from build123d import *

# Parameters (mm, degrees)
BOSS_EXTRUDE2_DEPTH = 5
CUT_EXTRUDE1_REACH  = 24.845
SKETCH3_R           = 2.1
CUT_EXTRUDE2_START  = -1.2
CUT_EXTRUDE2_DEPTH  = 3.6


with BuildPart() as part:
    # Sketch1 → Boss-Extrude2 (new body)
    with BuildSketch(Plane(origin=(0, 0, 0), x_dir=(1, 0, 0), z_dir=(0, 1, 0))):
        with BuildLine():
            Line((-0.939692556, 20.223890242), (-7.329602442, 2.667757118))
            ThreePointArc((-7.329602442, 2.667757118), (0, -7.8), (7.329602442, 2.667757118))
            Line((7.329602442, 2.667757118), (0.939692556, 20.223890242))
            ThreePointArc((0.939692556, 20.223890242), (0, 20.881870053), (-0.939692556, 20.223890242))
        make_face()
    extrude(amount=BOSS_EXTRUDE2_DEPTH)

    # Sketch3 → Cut-Extrude1 (cut, up to next)
    with BuildSketch(Plane(origin=(0, 5, 0), x_dir=(1, 0, 0), z_dir=(0, 1, 0)), mode=Mode.PRIVATE) as cut_extrude1_sk1:
        with Locations(Location((0, 0, 0), (0, 0, 270))):
            Circle(SKETCH3_R)
    cut_extrude1_tool1 = extrude(cut_extrude1_sk1.sketch, amount=-CUT_EXTRUDE1_REACH, mode=Mode.PRIVATE) & part.part
    add(cut_extrude1_tool1.solids().sort_by_distance((0, 5, 0))[0], mode=Mode.SUBTRACT)

    # Sketch4 → Cut-Extrude2 (cut)
    with BuildSketch(Plane(origin=(0, 5, 0), x_dir=(1, 0, 0), z_dir=(0, 1, 0)).offset(CUT_EXTRUDE2_START)):
        Polygon((0, 4.272391992), (-3.7, 2.136195996), (-3.7, -2.136195996), (0, -4.272391992), (3.7, -2.136195996), (3.7, 2.136195996), align=None)
    extrude(amount=-CUT_EXTRUDE2_DEPTH, mode=Mode.SUBTRACT)


solid = part.part
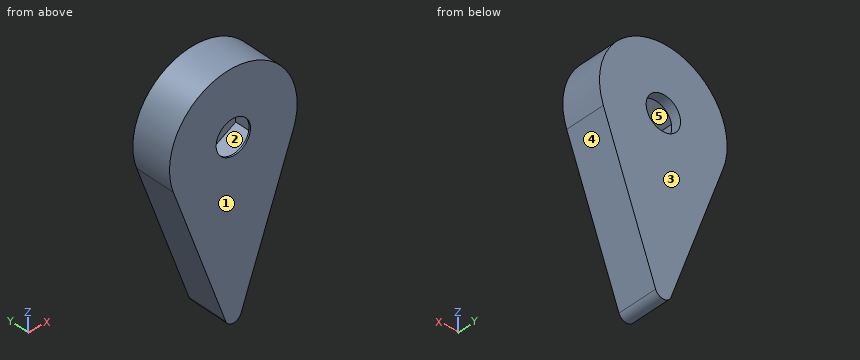
Work out the finished part from the listing and answer in its coordinate system (mm). Face numbers are marked on the shaded views. A direction names the side the tool comes from. Give positions to 0.01 mm unless a question says otherwise; leave off trailing zeros. Write each loop counter-clockwise with the first axis right and the second up, starting at its lowest first coordinate (ties: lowest second). Pieces come first, ordered by that corner, then holes. Notation, with made-up numbers: M -16.75,61.25 L 40.25,61.25 A22 ccw 40.25,78.25 Z; hole C 48,32.25 d3. An arc over 180 degrees is marked long. Answer as CSV lines item,"result".
Q1. A tool of negligible diameter and unlimited length cuts with its end or side. For the marked faces 1 and 2, from which of +Z, -Z, +X, -X, +Y, -Y can it reach the whole face along a straight path? Write none if from no direction.
A:
face 1,"+Z, -Z, +X, -X, -Y"
face 2,"none"
Q2. A cutting plane is placed at D-D on y = 4.6. Write down the section's boundary in (x, z).
A:
outline,"M -7.33,-2.67 L -0.94,-20.22 A1 ccw 0.94,-20.22 L 7.33,-2.67 A7.8 ccw long Z; hole C 0,0 d4.2"
Q3. Given P1, Ø4, axis at x = 0, z = 0, coming from the -Y side; P2, Ø2, axis at x = -4.5, y = 1.5, coming from the +Z side, each flat-ended and moving along its own axis, determine where each tip first touches the part or whether it passes through.
A:
P1,"passes through"
P2,"stops at z = 6.97"
Q4. A cutting plane is placed at C-C on x = 1.5. Write down the section's boundary in (y, z).
A:
outline,"M 0,-18.68 L 5,-18.68 L 5,-1.47 L 3.8,-1.47 L 3.8,-3.41 L 0.2,-3.41 L 0.2,-1.47 L 0,-1.47 Z; M 0,1.47 L 0.2,1.47 L 0.2,3.41 L 3.8,3.41 L 3.8,1.47 L 5,1.47 L 5,7.65 L 0,7.65 Z"
Q5. A cutting plane is placed at B-B on z = 0. Write down the section's boundary in (x, y), plus the area to 3 significant figures.
A:
outline,"M -7.8,0 L -2.1,0 L -2.1,0.2 L -3.7,0.2 L -3.7,3.8 L -2.1,3.8 L -2.1,5 L -7.8,5 Z; M 2.1,0 L 7.8,0 L 7.8,5 L 2.1,5 L 2.1,3.8 L 3.7,3.8 L 3.7,0.2 L 2.1,0.2 Z"
area,"45.5 mm²"
Q6. Find the intervals of material crossed by probe 1 along X at (y, z) = (0.15, 0); probe 2 along Y at (x, z) = (2.75, 2.5); probe 3 along X at (y, z) = (2, 4), in increasing order. Write a range as [from, to].
A:
probe 1,"x = [-7.8, -2.1], [2.1, 7.8]"
probe 2,"y = [0, 0.2], [3.8, 5]"
probe 3,"x = [-6.7, -0.47], [0.47, 6.7]"
Q7. A cutting plane is placed at A-A on y = 2.8. Write down the section's boundary in (x, z), plus the area to 3 significant figures.
A:
outline,"M -7.33,-2.67 L -0.94,-20.22 A1 ccw 0.94,-20.22 L 7.33,-2.67 A7.8 ccw long Z; hole M -3.7,-2.14 L 0,-4.27 L 3.7,-2.14 L 3.7,2.14 L 0,4.27 L -3.7,2.14 Z"
area,"235 mm²"
Q8. The mould has two halves that part along Z. Classify the marked faces 3, 4 and 5: +Z half, -Z half, draft (parallel to the pull), parting line (faces both ways), or undercut.
A:
face 3,"draft"
face 4,"-Z half"
face 5,"undercut"
